from build123d import *

# Parameters (mm, degrees)
SKETCH_1_R          = 8
SKETCH_1_R_2        = 5
EXTRUDE_1_DEPTH     = 20
CUT_EXTRUDE_2_DEPTH = 9.5
CUT_EXTRUDE_3_DEPTH = 4


with BuildPart() as part:
    # Эскиз1 → Вытянуть1 (new body)
    with BuildSketch(Plane(origin=(0, 0, 0), x_dir=(1, 0, 0), z_dir=(0, 1, 0))):
        with Locations(Location((0, 0, 0), (0, 0, 270))):
            Circle(SKETCH_1_R)
        with Locations(Location((0, 0, 0), (0, 0, 270))):
            Circle(SKETCH_1_R_2, mode=Mode.SUBTRACT)
    extrude(amount=EXTRUDE_1_DEPTH)

    # Эскиз2 → Вытянуть2 (cut)
    with BuildSketch(Plane(origin=(0, 20, 0), x_dir=(1, 0, 0), z_dir=(0, 1, 0))):
        with BuildLine():
            Line((-6, 1.5), (6, 1.5))
            ThreePointArc((6, 1.5), (6.184658438, 0), (6, -1.5))
            Line((6, -1.5), (-6, -1.5))
            ThreePointArc((-6, -1.5), (-6.184658438, 0), (-6, 1.5))
        make_face()
    extrude(amount=-CUT_EXTRUDE_2_DEPTH, mode=Mode.SUBTRACT)

    # Эскиз4 → Вырез-Повернуть2 (revolve, cut)
    with BuildSketch(Plane.XY, mode=Mode.PRIVATE) as cut_revolve_2_sk:
        Polygon((0, 10.5), (6, 10.5), (6.184658438, 10.5), (6.184658438, 13.5), (6, 13.5), (0, 13.5), align=None)
    revolve(cut_revolve_2_sk.sketch.rotate(Axis((0, 0, 0), (0, 1, 0)), 270), axis=Axis((0, 0, 0), (0, 1, 0)), mode=Mode.SUBTRACT)

    # Эскиз5 → Вытянуть3 (cut)
    with BuildSketch(Plane.XZ.offset(-13.5)):
        Polygon((-1.5, 6.184658438), (1.5, 6.184658438), (1.5, 6), (1.5, -6), (1.5, -6.184658438), (-1.5, -6.184658438), (-1.5, -6), (-1.5, 6), align=None)
    extrude(amount=-CUT_EXTRUDE_3_DEPTH, mode=Mode.SUBTRACT)


solid = part.part
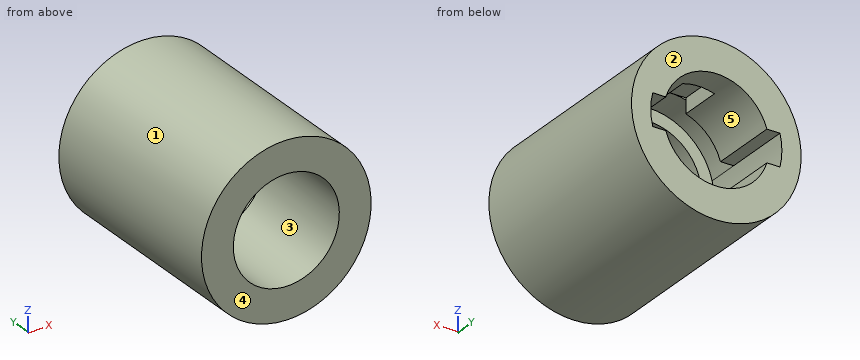
Source: CAD feature listing. Evaluate the final solid. Frame: model axes, mm. Face numbers are marked on the shaded views. A direction names the side the tool comes from. Give positions to 0.01 mm unless a question says otherwise; leave off trailing zeros. Write each loop counter-clockwise with the first axis right and the second up, starting at its lowest first coordinate (ties: lowest second). Pieces come first, ordered by that corner, then holes. Notation, with made-up numbers: M -7.75,7 L 13.25,7 A37 ccw 13.25,46 Z; hole C 4.5,50 d4. An arc over 180 degrees is marked long. Return JSON: item names as keys, results as strings. Group by question number.
1) First-contact query: pin 1 Ø8 at (x, y) = (5.5, 17) entering from +Z; pin 2 Ø1 at (x, y) = (-5, 17) entering from +Z; pin 3 Ø6 at (y, z) = (5, 4.5) entering from -X. Flat tips, straight axial feed; report the tip coordinate or a pass-through.
2) Cut plane A-A, the plane z = 0. Output: boundary loops of the cut face in (x, y).
3) Cut plane B-B, the plane y = 18. Output: boundary loops of the cut face in (x, z), then the cut area to 3 significant figures.
4) Set-up query: the marked faces 4 and 5. Return all of +Z, -Z, +X, -X, +Y, -Y with unobstructed straight access to the full face (end or side cutting, diameter ignored); none if empty.
5) Cut plane C-C, the plane x = 2.75. Output: boundary loops of the cut face in (y, z).
6) Draft query along X for the marked faces 1, 2 and 3. Return one class per face: released by +X, released by -X, zero draft, split by the parting line, or undercut.
7) Ray query, L1, parallel to Y at x = 3, z = 4.5; L2, parallel to X at y = 3.75, z = 0; L3, parallel to X at y = 12.25, z = 1.25. Return the intervals inside material, ascending.
8) Cut plane D-D, the plane z = -5.25. Output: boundary loops of the cut face in (x, y).
Data:
{
 "1": {"pin 1": "stops at z = 7.86", "pin 2": "stops at z = 6.61", "pin 3": "stops at x = -7.86"},
 "2": {"outline": "M -8,0 L -5,0 L -5,10.5 L -6.18,10.5 L -6.18,20 L -8,20 Z; M 5,0 L 8,0 L 8,20 L 6.18,20 L 6.18,10.5 L 5,10.5 Z"},
 "3": {"outline": "C 0,0 d16; hole M -6,-1.5 L -4.77,-1.5 A5 ccw 4.77,-1.5 L 6,-1.5 A6.18 ccw 6,1.5 L 4.77,1.5 A5 ccw -4.77,1.5 L -6,1.5 A6.18 ccw Z", "area": "115 mm²"},
 "4": {"face 4": "+Z, -Z, +X, -X, -Y", "face 5": "+Y, -Y"},
 "5": {"outline": "M 0,-7.51 L 20,-7.51 L 20,-4.18 L 13.5,-4.18 L 13.5,-5.54 L 10.5,-5.54 L 10.5,-4.18 L 0,-4.18 Z; M 0,4.18 L 10.5,4.18 L 10.5,5.54 L 13.5,5.54 L 13.5,4.18 L 20,4.18 L 20,7.51 L 0,7.51 Z"},
 "6": {"face 1": "split by the parting line", "face 2": "zero draft", "face 3": "undercut"},
 "7": {"L1": "y = 0 to 10.5, 13.5 to 20", "L2": "x = -8 to -5, 5 to 8", "L3": "x = -7.9 to -6.06, 6.06 to 7.9"},
 "8": {"outline": "M -6.04,0 L 6.04,0 L 6.04,20 L -6.04,20 Z; hole M -3.27,10.5 L 3.27,10.5 L 3.27,13.5 L 1.5,13.5 L 1.5,17.5 L -1.5,17.5 L -1.5,13.5 L -3.27,13.5 Z"}
}
